Autodesk Inventor part; units mm, degrees
ref_plane "YZ Plane" through (0, 0, 0) normal (1, 0, 0) x (0, 1, 0)
ref_plane "XZ Plane" through (0, 0, 0) normal (0, 1, 0) x (-1, 0, 0)
ref_plane "XY Plane" through (0, 0, 0) normal (0, 0, 1) x (1, 0, 0)
sketch "Sketch1" plane through (0, 0, 0) normal (0, 0, 1) x (1, 0, 0)
  line L0 (0, 0) -> (0, 54.375) construction
  line L1 (0, 54.375) -> (192, 54.375)
  line L2 (0, 0) -> (524.135, 0) construction
  line L3 (254.7886, 18.124) -> (254.7886, 0) construction
  line L4 (192, 54.375) -> (254.7886, 18.124)
  line L5 (254.7886, 18.124) -> (325.1228, 36.97)
  line L6 (325.1228, 36.97) -> (325.1228, 0) construction
  line L7 (192, 54.375) -> (192, 0) construction
  line L8 (325.1228, 51.4639) -> (256.7665, 33.1479)
  line L9 (256.7665, 33.1479) -> (195.7513, 68.375)
  line L10 (195.7513, 68.375) -> (0, 68.375)
  line L11 (0, 54.375) -> (0, 68.375)
  line L12 (325.1228, 36.97) -> (325.1228, 51.4639)
  line L13 (195.7513, 68.375) -> (195.7513, 78.375)
  line L14 (195.7513, 78.375) -> (186.3124, 78.375)
  line L15 (186.3124, 78.375) -> (186.3124, 68.375)
  dimension "d0" = 54.375
  dimension "d1" = 192
  dimension "d2" = 18.124
  dimension "d3" = 30
  dimension "d4" = 15
  dimension "d5" = 36.97
  dimension "d6" = 14
  dimension "d12" = 10
revolve "Revolution1" add sketch "Sketch1" angle 360 about axis through (0, 0, 0) along (1, 0, 0) contours L11 L10 L9 L8 L12 L5 L4 L1
sketch "Sketch2" plane through (0, 0, 0) normal (-1, 0, 0) x (0, 0, 1)
  circle A0 centre (0, 0) radius 61.375 construction
  circle A1 centre (0, 61.375) radius 3
  dimension "d8" = 122.75
  dimension "d9" = 6
extrude "Extrusion1" cut sketch "Sketch2" against normal blind 192
properties part number "concept3" material "Aluminum 6061"
The model under review builds one solid part; all positions refer to its coordinate system, in mm. A direction names the side the tool comes from. Give positions to 0.01 mm unless a question says otherwise; leave off trailing zeros. Write each loop counter-clockwise with the first axis right and the second up, starting at its lowest first coordinate (ties: lowest second). Pieces come first, ordered by that corner, then holes.
1. Draft analysis for pull direction Y (two halves, no side actions). For faces 4 (the conical face through (246.17, -8.512, 38.332)), 5 (the cylindrical face through (97.34, -11.79, -53.08)), 6 (the flat face through (0, -21, 51)), state which applies: +Y half, -Y half, draft (parallel to the pull), parting line (faces both ways), or undercut.
2. Tool access review of faces 1 (the flat face through (192, 61, 0)), 2 (the conical face through (282.633, -3.331, 25.367)), 3 (the conical face through (283.828, 38.533, 12.135)): name each direction out of +Z, -Z, +X, -X, +Y, -Y from which nothing blocks a thin tool from reaching the whole face with its end or side.
3. Add section B-B, the plane x = 238. Write out the cut boundary in (y, z).
4. Wall thickness on L1, parallel to Z at x = 131, y = 0 (3 decimals); L2, parallel to Z at x = 199, y = -30; L3, parallel to Y at x = 116, z = 21.5: over which ranges is each line inside the solid? List them lowest first.
5. Add section A-A, the plane y = 0. Write out the cut boundary in (x, z) (1 decimal), plus the area to 3 significant figures.
6. For P1, Ø4, axis at x = 92, y = 48, coming from the +Z side; P2, Ø10, axis at y = 34, z = 0.5, coming from the +X side; P3, Ø2, axis at x = 132, z = 23, coming from the +Y side; P4, Ø1.5, axis at x = 235.5, z = -17.5, coming from the +Y side, all flat-tipped, find the tip position at first contact; note any pin that passes through.
7. Add section D-D, the plane x = 286.5. Write out the cut boundary in (y, z), plus the area to 3 significant figures.
8. Add section C-C, the plane x = 180.5. Write out the cut boundary in (y, z) (3 decimals).
Worked answers:
1. face 4: parting line
1. face 5: undercut
1. face 6: draft
2. face 1: -X
2. face 2: +X
2. face 3: none
3. outline: circle Ø87.97 at (0, 0); hole circle Ø55.63 at (0, 0)
4. L1: z = -68.375 to -54.375, 54.375 to 68.375
4. L2: z = -59.35 to -40.42, 40.42 to 59.35
4. L3: y = -64.91 to -49.94, 49.94 to 64.91
5. outline: (0, -68.4) - (195.8, -68.4) - (256.8, -33.1) - (325.1, -51.5) - (325.1, -37) - (254.8, -18.1) - (192, -54.4) - (0, -54.4) - close; (0, 54.4) - (192, 54.4) - (254.8, 18.1) - (325.1, 37) - (325.1, 51.5) - (256.8, 33.1) - (195.8, 68.4) - (0, 68.4) - close
5. area: 9,440 mm2
6. P1: stops at z = 50.59
6. P2: stops at x = 325.12
6. P3: stops at y = 64.74
6. P4: stops at y = 42.48
7. outline: circle Ø82.23 at (0, 0); hole circle Ø53.24 at (0, 0)
7. area: 3,080 mm2
8. outline: circle Ø136.75 at (0, 0); hole circle Ø108.75 at (0, 0); hole circle Ø6 at (61.375, 0)
